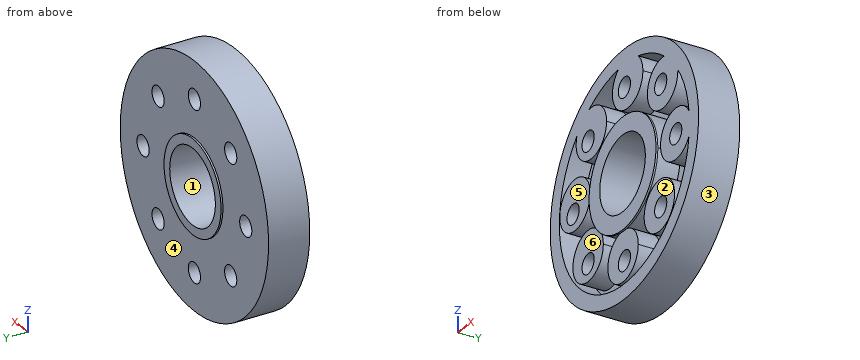
```python
from build123d import *

# Parameters (mm, degrees)
CROQUIS1_R              = 9.75
CROQUIS1_R_2            = 3
CROQUIS1_R_3            = 0.8
SALIENTE_EXTRUIR1_DEPTH = 1.65
CROQUIS1_3_R            = 3.75
CROQUIS1_3_R_2          = 3
SALIENTE_EXTRUIR2_DEPTH = 1.8
CROQUIS2_R              = 2
CORTAR_EXTRUIR3_DEPTH   = 1.8
CROQUIS3_R              = 4.4
CROQUIS3_R_2            = 3
SALIENTE_EXTRUIR3_DEPTH = 0.15


with BuildPart() as part:
    # Croquis1 → Saliente-Extruir1 (new body, symmetric)
    with BuildSketch(Plane(origin=(0, 0, 0), x_dir=(1, 0, 0), z_dir=(0, 1, 0))):
        Circle(CROQUIS1_R)
        Circle(CROQUIS1_R_2, mode=Mode.SUBTRACT)
        with Locations((6.75, 0)):
            Circle(CROQUIS1_R_3, mode=Mode.SUBTRACT)
        with Locations((0, -6.75)):
            Circle(CROQUIS1_R_3, mode=Mode.SUBTRACT)
        with Locations((-6.75, 0)):
            Circle(CROQUIS1_R_3, mode=Mode.SUBTRACT)
        with Locations((0, 6.75)):
            Circle(CROQUIS1_R_3, mode=Mode.SUBTRACT)
        with Locations((4.772970773, -4.772970773)):
            Circle(CROQUIS1_R_3, mode=Mode.SUBTRACT)
        with Locations((-4.772970773, -4.772970773)):
            Circle(CROQUIS1_R_3, mode=Mode.SUBTRACT)
        with Locations((-4.772970773, 4.772970773)):
            Circle(CROQUIS1_R_3, mode=Mode.SUBTRACT)
        with Locations((4.772970773, 4.772970773)):
            Circle(CROQUIS1_R_3, mode=Mode.SUBTRACT)
    extrude(amount=SALIENTE_EXTRUIR1_DEPTH, both=True)

    # Croquis1_3 → Saliente-Extruir2 (add, symmetric)
    with BuildSketch(Plane(origin=(0, 0, 0), x_dir=(1, 0, 0), z_dir=(0, 1, 0))):
        Circle(CROQUIS1_3_R)
        Circle(CROQUIS1_3_R_2, mode=Mode.SUBTRACT)
    extrude(amount=SALIENTE_EXTRUIR2_DEPTH, both=True)

    # Croquis2 → Cortar-Extruir3 (cut)
    with BuildSketch(Plane.XZ.offset(1.65)):
        with BuildLine():
            ThreePointArc((8.493703704, -0.979539378), (4.75, 0), (8.493703704, 0.979539378))
            ThreePointArc((8.493703704, 0.979539378), (7.998376267, 3.021336972), (7.02006773, 4.880691454))
            ThreePointArc((7.02006773, 4.880691454), (7.02224488, 4.826850669), (7.022970773, 4.772970773))
            ThreePointArc((7.022970773, 4.772970773), (3.536549224, 3.434856062), (5.232419794, 6.761973314))
            ThreePointArc((5.232419794, 6.761973314), (3.619603246, 7.746029457), (1.830044014, 8.351852424))
            ThreePointArc((1.830044014, 8.351852424), (2.27157135, 7.69926144), (2.426776695, 6.926776695))
            ThreePointArc((2.426776695, 6.926776695), (-0.457693454, 5.132978336), (-0.79093586, 8.513337798))
            ThreePointArc((-0.79093586, 8.513337798), (-2.79976514, 8.078602303), (-4.646803784, 7.177026863))
            ThreePointArc((-4.646803784, 7.177026863), (-3.042587429, 6.716523558), (-2.346194078, 5.199747468))
            ThreePointArc((-2.346194078, 5.199747468), (-4.673942073, 3.226784911), (-6.238775329, 5.846381992))
            ThreePointArc((-6.238775329, 5.846381992), (-3.594367278, -7.757771837), (8.493703704, -0.979539378))
        make_face()
        with BuildLine():
            ThreePointArc((0.327362602, -4.387805115), (1.405670554, -5.100169462), (1.823223305, -6.323223305))
            ThreePointArc((1.823223305, -6.323223305), (-1.443575646, -7.870873271), (-0.571997114, -4.362661951))
            ThreePointArc((-0.571997114, -4.362661951), (-1.892548808, -3.972185671), (-3.027723734, -3.192630419))
            ThreePointArc((-3.027723734, -3.192630419), (-2.837706698, -3.6646868), (-2.772970773, -4.169417382))
            ThreePointArc((-2.772970773, -4.169417382), (-6.562508569, -5.062476438), (-3.57052525, -2.571254448))
            ThreePointArc((-3.57052525, -2.571254448), (-1.350868035, 4.187499917), (4.4, 0))
            ThreePointArc((4.4, 0), (3.224933755, -2.993292882), (0.327362602, -4.387805115))
        make_face(mode=Mode.SUBTRACT)
        with Locations((4.596194078, -4.596194078)):
            Circle(CROQUIS2_R, mode=Mode.SUBTRACT)
        with Locations((-6.5, 0.603553391)):
            Circle(CROQUIS2_R, mode=Mode.SUBTRACT)
    extrude(amount=-CORTAR_EXTRUIR3_DEPTH, mode=Mode.SUBTRACT)

    # Croquis3 → Saliente-Extruir3 (add)
    with BuildSketch(Plane.XZ.offset(1.65)):
        Circle(CROQUIS3_R)
        Circle(CROQUIS3_R_2, mode=Mode.SUBTRACT)
    extrude(amount=SALIENTE_EXTRUIR3_DEPTH)


solid = part.part
```
Can you work these out from the model? Positions are in its coordinate system, mm. Face numbers are marked on the shaded views. A direction names the side the tool comes from. Give positions to 0.01 mm unless a question says otherwise; leave off trailing zeros. Order: outer loops, then holes, each group sorted by start corner. A loop starts at its lowest first (then second) coordinate and runs counter-clockwise, first axis right, second up. Notation, with made-up numbers: M 43,40.5 L 100,40.5 A16 cw 100,49.5 Z; hole C 49.5,22.5 d4. An arc over 180 degrees is marked long. Write item = value, one per line. Start each with the question number.
Q1. Suppose I cut it at B-B (x = 1.5). Write out the boundary of the cut face in (y, z), plus the area to 3 significant figures.
Q2. I need wall thicknesses on probe 1 along Z at (x, y) = (0, 0.05); probe 2 along Z at (x, y) = (-5, 1.4); probe 3 along Z at (x, y) = (5.25, 0.65). Which ranges of each line are inside material? Lowest first, please. Write a range as [from, to].
Q3. We'd pull the mould along Z, two halves only. Please class the marked faces 1, 2 and 3: pulls with the +Z half, pulls with the -Z half, needs draft (parallel to the pull), parting line crosses it, or undercut.
Q4. Suppose I cut it at A-A (y = -0.65). Count the separate pieces of the cut face and the enclosed holes in it, plus the area to 3 significant figures.
Q5. For the marked faces 4, 5 and 6, which set-ups out of +Z, -Z, +X, -X, +Y, -Y let a thin tool reach every point of the face, with its end or its side?
Q6. Will these pins go through, and if not, where does the flat tip stop? pin 1 Ø2 at (x, z) = (0, 6.75) entering from +Y; pin 2 Ø2 at (x, y) = (-4, 0.5) entering from -Z; pin 3 Ø1.8 at (x, z) = (0, -6.75) entering from -Y.
Check result:
q1.outline = M -1.8,-4.14 L 0.15,-4.14 L 0.15,-5.23 L -1.65,-5.23 L -1.65,-7.41 L 0.15,-7.41 L 0.15,-8.42 L -1.65,-8.42 L -1.65,-9.63 L 1.65,-9.63 L 1.65,-3.44 L 1.8,-3.44 L 1.8,-2.6 L -1.8,-2.6 Z; M -1.8,2.6 L 1.8,2.6 L 1.8,3.44 L 1.65,3.44 L 1.65,9.63 L -1.65,9.63 L -1.65,5.24 L 0.15,5.24 L 0.15,4.14 L -1.8,4.14 Z
q1.area = 41.4 mm2
q2.probe_1 = [-9.75, -8.55], [-8.32, -7.55], [-5.95, -3], [3, 4.4], [4.97, 5.95], [7.55, 9.75]
q2.probe_2 = [-8.37, -5.54], [-4.01, 4.01], [5.54, 8.37]
q2.probe_3 = [-8.22, -5.42], [-4.13, 4.13], [5.42, 8.22]
q3.face_1 = undercut
q3.face_2 = needs draft
q3.face_3 = parting line crosses it
q4.separate_pieces = 4
q4.enclosed_holes = 10
q4.area = 184 mm2
q5.face_4 = +Y
q5.face_5 = +Z, -Z, -X, -Y
q5.face_6 = -Z, -X, -Y
q6.pin_1 = 1.65
q6.pin_2 = -9.28
q6.pin_3 = -1.65
